Autodesk Inventor part; units mm, degrees
ref_plane "YZ Plane" through (0, 0, 0) normal (1, 0, 0) x (0, 1, 0)
ref_plane "XZ Plane" through (0, 0, 0) normal (0, 1, 0) x (-1, 0, 0)
ref_plane "XY Plane" through (0, 0, 0) normal (0, 0, 1) x (1, 0, 0)
sketch "Sketch1" plane through (0, 0, 0) normal (0, 1, 0) x (-1, 0, 0)
  circle A0 centre (30.1, 6) radius 2.1
  circle A1 centre (49.9, 6) radius 2.1
  line L0 (0, 0) -> (80, 0)
  line L1 (80, 0) -> (80, 12)
  line L2 (0, 12) -> (80, 12)
  line L3 (0, 0) -> (0, 12)
  line L4 (40, 12) -> (15, 12)
  line L5 (15, 12) -> (15, 0)
  line L6 (15, 0) -> (65, 0)
  line L7 (65, 0) -> (65, 12)
  circle A2 centre (49.9, 6) radius 2.75
  circle A3 centre (30.1, 6) radius 2.75
  dimension "d0" = 25
  dimension "d1" = 50
  dimension "d2" = 5.5
  dimension "d3" = 5.5
extrude "Extrusion1" add sketch "Sketch1" along normal blind 3 contours L5 L2 L7 L0
sketch "Sketch2" plane through (0, 3, 0) normal (0, 1, 0) x (1, 0, 0)
  line L0 (-15, -12) -> (-15, 0)
  line L1 (-65, 0) -> (-65, -12)
  line L2 (-15, -12) -> (-65, -12)
  line L3 (-65, -12) -> (-65, -9.9998)
  line L4 (-65, -9.9998) -> (-15, -9.9998)
  line L5 (-15, -9.9998) -> (-15, -12)
  point P0 (0, 0)
extrude "Extrusion2" add sketch "Sketch2" along normal blind 7
sketch "Sketch3" plane through (-15, 3, 9.9998) normal (0, 0, -1) x (-1, 0, 0)
  line L0 (0, -3) -> (0, 7)
  line L1 (0, -0.0684) -> (30, -0.0684)
  line L2 (0, -0.0684) -> (30, -0.0684) construction
  line L3 (30, -0.0684) -> (30, 3.4316)
  line L4 (30, 3.4316) -> (40, 3.4316)
  line L5 (40, 3.4316) -> (20, 3.4316)
  circle A0 centre (20, 3.4316) radius 1.5
  circle A1 centre (40, 3.4316) radius 1.5
  point P0 (-15, -3)
  dimension "d8" = 30
  dimension "d9" = 0
  dimension "d10" = 3.5
  dimension "d11" = 10
  dimension "d12" = 20
  dimension "d13" = 3
  dimension "d14" = 3
extrude "Extrusion3" cut sketch "Sketch3" against normal blind 10
sketch "Sketch4" plane through (-15, 0, 12) normal (1, 0, 0) x (0, 0, -1)
  line L0 (0, 0) -> (12, 0)
  line L1 (12, 0) -> (12, 3)
  line L2 (2.0002, 3) -> (12, 3)
  line L3 (2.0002, 3) -> (2.0002, 10)
  line L4 (0, 10) -> (2.0002, 10)
  line L5 (0, 0) -> (0, 10)
extrude "Extrusion4" cut sketch "Sketch4" against normal blind 10
sketch "Sketch5" plane through (-65, 0, 0) normal (-1, 0, 0) x (0, 0, 1)
  line L0 (8.75, 3) -> (8.75, 0)
  line L1 (0, 0) -> (12, 0)
  line L2 (12, 0) -> (12, 10)
  line L3 (9.9998, 10) -> (12, 10)
  line L4 (9.9998, 3) -> (9.9998, 10)
  line L5 (0, 3) -> (9.9998, 3)
  line L6 (0, 0) -> (0, 3)
extrude "Extrusion5" cut sketch "Sketch5" against normal blind 5
properties part number "end_button"
Verification items for the finished model (mm, model axes). A direction names the side the tool comes from. Coordinates: 2 decimals unless noted, no trailing zeros. Write each loop counter-clockwise with the first axis right and the second up, starting at its lowest first coordinate (ties: lowest second). Pieces come first, ordered by that corner, then holes. Notation, with made-up numbers: M 13.25,16 L 42.25,16 A3 cw 42.25,21 Z; hole C 5.5,20 d6. An arc over 180 degrees is marked long. Answer as a JSON object with one key per item and string values. Group by question number.
(1) Cross-section at D-D, the plane x = -55. Record the cut outline in (y, z), and give its area (3 significant figures).
(2) Gauge pin test, flat ends, axial feed: pin 1 (1 mm diameter, centred on x = -56.5, z = 7.5, fed in from +Y); pin 2 (5 mm diameter, centred on x = -55, y = 6.43, fed in from -Z). Record the tip position at first contact, or that the pin passes through.
(3) Cross-section at B-B, the plane z = 6. Record the cut outline in (x, y).
(4) Cross-section at A-A, the plane x = -30.1. Record the cut outline in (y, z), and give its area (3 significant figures).
(5) Tool access check on faces 1 (the face through (-43, 6, 10)), 2 (the face through (-56.43, 6.88, 10.99)). Record the directions out of +Z, -Z, +X, -X, +Y, -Y that give a thin tool (end or side, any length) a straight path to the whole face; none if there is none.
(6) Release check for a two-part mould opening along Z. For faces 3 (the face through (-27.353, 1.479, 5.879)), 4 (the face through (-42, 5, 12)), 5 (the face through (-52.44, 1.48, 7.05)), 6 (the face through (-42, 3, 5)) record: +Z half, -Z half, draft (parallel to the pull), parting line (faces both ways), or undercut.
(7) Material ranges on line 1 (Y direction, x = -35, z = 11); line 2 (X direction, y = 2.75, z = 7.5); line 3 (X direction, y = 1.75, z = 5), recorded low to high.
(8) Cross-section at C-C, the plane y = 6. Record the cut outline in (x, z), and give its area (3 significant figures).
Reply:
{
 "1": {"outline": "M 0,0 L 3,0 L 3,10 L 4.93,10 L 4.93,12 L 0,12 Z; M 7.93,10 L 10,10 L 10,12 L 7.93,12 Z", "area": "44.0 mm²"},
 "2": {"pin 1": "y = 3", "pin 2": "z = 10"},
 "3": {"outline": "M -60,0 L -52.65,0 L -52.65,3 L -60,3 Z; M -47.15,0 L -32.85,0 L -32.85,3 L -47.15,3 Z; M -27.35,0 L -25,0 L -25,3 L -27.35,3 Z"},
 "4": {"outline": "M 0,0 L 3,0 L 3,3.25 L 0,3.25 Z; M 0,8.75 L 3,8.75 L 3,10 L 10,10 L 10,12 L 0,12 Z", "area": "33.5 mm²"},
 "5": {"face 1": "-Z, +X, -X, +Y", "face 2": "+Z, -Z"},
 "6": {"face 3": "undercut", "face 4": "+Z half", "face 5": "undercut", "face 6": "draft"},
 "7": {"line 1": "0 to 4.93, 7.93 to 10", "line 2": "-60 to -52.2, -47.6 to -32.4, -27.8 to -25", "line 3": "-60 to -52.46, -47.34 to -32.66, -27.54 to -25"},
 "8": {"outline": "M -60,10 L -56.44,10 L -56.44,12 L -60,12 Z; M -53.56,10 L -36.44,10 L -36.44,12 L -53.56,12 Z; M -33.56,10 L -25,10 L -25,12 L -33.56,12 Z", "area": "58.5 mm²"}
}
